Could you check a few things on this model? Use its own coordinates, in mm. A direction names the side the tool comes from. Coordinates: 2 decimals unless noted, no trailing zeros. Order: outer loops, then holes, each group sorted by start corner. A loop starts at its lowest first (then second) coordinate and runs counter-clockwise, first axis right, second up. Notation, with made-up numbers: (27, 54) - (67, 54) arc R16 cw to (67, 67) - close; hole circle Ø3 at (14, -8.75). An arc over 180 degrees is marked (long way). One line per item, written item: value. Start each with the question number.
from build123d import *

# Parameters (mm, degrees)
ESQUISSE1_W                     = 150
ESQUISSE1_H                     = 50
BOSS_EXTRU_1_DEPTH              = 10
ESQUISSE2_R                     = 5
BOSS_EXTRU_2_DEPTH              = 50
R_P_TITION_LIN_AIRE1_COUNT      = 5
R_P_TITION_LIN_AIRE1_PITCH      = 32
R_P_TITION_LIN_AIRE1_COUNT_DIR2 = 3
R_P_TITION_LIN_AIRE1_PITCH_DIR2 = 13


with BuildPart() as part:
    # Esquisse1 → Boss.-Extru.1 (new body)
    with BuildSketch(Plane(origin=(0, 0, 0), x_dir=(1, 0, 0), z_dir=(0, 1, 0))):
        Rectangle(ESQUISSE1_W, ESQUISSE1_H)
    extrude(amount=BOSS_EXTRU_1_DEPTH)

    # Esquisse2 → Boss.-Extru.2 (add)
    with BuildSketch(Plane(origin=(0, 10, 0), x_dir=(1, 0, 0), z_dir=(0, 1, 0))):
        with Locations(Location((-65, -15, 0), (0, 0, 270))):
            Circle(ESQUISSE2_R)
    boss_extru_2 = extrude(amount=BOSS_EXTRU_2_DEPTH)

    # Répétition linéaire1: Boss.-Extru.2 5 × 3
    with Locations(*[(i * R_P_TITION_LIN_AIRE1_PITCH, 0, -j * R_P_TITION_LIN_AIRE1_PITCH_DIR2) for i in range(R_P_TITION_LIN_AIRE1_COUNT) for j in range(R_P_TITION_LIN_AIRE1_COUNT_DIR2) if (i, j) != (0, 0)]):
        add(boss_extru_2)


solid = part.part
Q1. I want a section at B-B on z = 2. Please give me the cut outline in (x, y).
Q2. If I drill on L1, parallel to X at y = 54.5, z = 1.5; L2, parallel to Z at x = 66, y = 46; L3, parallel to Z at x = -29, y = 38, over which ranges is the centre line in solid material (lowest first)?
Q3. I want a section at D-D on z = -10.5. Please give me the cut outline in (x, y).
Q4. We'd pull the mould along Z, two halves only. Please class faces 3 (the flat face through (-1, 0, 0)), 4 (the cylindrical face through (67.957, 34.65, 14.349)), 5 (the cylindrical face through (-37.88, 34.65, 13.92)), 6 (the flat face through (-1, 5, 25)): +Z half, -Z half, draft (parallel to the pull), parting line (faces both ways), or undercut.
Q5. Which directions (+Z, -Z, +X, -X, +Y, -Y) give clear straight access to the entire face, cutting with the end or side of a thin tool? Please do faces 1 (the flat face through (63, 60, 2)), 2 (the cylindrical face through (-61, 35, -8)).
Q6. I want a section at A-A on y = 46. State how many separate pieces and enclosed holes the cut face has, then the cut area to 3 significant figures.
Q7. I want a section at C-C on x = 63. Please give me the cut outline in (y, z), then the cut area to 3 significant figures.
Q8. I'm going to push flat-ended pins straight in: pin 1 (3 mm diameter, centred on y = 47.5, z = -6, fed in from -X); pin 2 (6 mm diameter, centred on y = 36, z = 1.5, fed in from +X). Where does each tip first touch, or does it pass through?
Values follow:
1. outline: (-75, 0) - (75, 0) - (75, 10) - (68, 10) - (68, 60) - (58, 60) - (58, 10) - (36, 10) - (36, 60) - (26, 60) - (26, 10) - (4, 10) - (4, 60) - (-6, 60) - (-6, 10) - (-28, 10) - (-28, 60) - (-38, 60) - (-38, 10) - (-60, 10) - (-60, 60) - (-70, 60) - (-70, 10) - (-75, 10) - close
2. L1: x = -69.97 to -60.03, -37.97 to -28.03, -5.97 to 3.97, 26.03 to 35.97, 58.03 to 67.97
2. L2: z = -15 to -7, -2 to 6, 11 to 19
2. L3: z = -14 to -8, -1 to 5, 12 to 18
3. outline: (-75, 0) - (75, 0) - (75, 10) - (67.97, 10) - (67.97, 60) - (58.03, 60) - (58.03, 10) - (35.97, 10) - (35.97, 60) - (26.03, 60) - (26.03, 10) - (3.97, 10) - (3.97, 60) - (-5.97, 60) - (-5.97, 10) - (-28.03, 10) - (-28.03, 60) - (-37.97, 60) - (-37.97, 10) - (-60.03, 10) - (-60.03, 60) - (-69.97, 60) - (-69.97, 10) - (-75, 10) - close
4. face 3: draft
4. face 4: undercut
4. face 5: undercut
4. face 6: +Z half
5. face 1: +Z, -Z, +X, -X, +Y
5. face 2: +Y
6. separate pieces: 15
6. enclosed holes: 0
6. area: 1,180 mm^2
7. outline: (0, -25) - (10, -25) - (10, -16) - (60, -16) - (60, -6) - (10, -6) - (10, -3) - (60, -3) - (60, 7) - (10, 7) - (10, 10) - (60, 10) - (60, 20) - (10, 20) - (10, 25) - (0, 25) - close
7. area: 2,000 mm^2
8. pin 1: stops at x = -68.57
8. pin 2: stops at x = 68
